from build123d import *

# Parameters (mm, degrees)
F0_W     = 260
F0_H     = 130
F1_DEPTH = 50
F2_R     = 50
F3_DEPTH = 10
F4_W     = 240
F4_H     = 110
F5_DEPTH = 30
F7_DEPTH = 260
F8_R     = 4
F8_R_2   = 4.17612
F9_DEPTH = 25


with BuildPart() as f1:
    # F0 (on Front) → F1 (new body)
    with BuildSketch(Plane.XZ):
        Rectangle(F0_W, F0_H)
    extrude(amount=F1_DEPTH)

    # F2 (on face) → F3 (cut)
    with BuildSketch(Plane(origin=(0, 0, 0), x_dir=(-1, 0, 0), z_dir=(0, 1, 0))):
        with Locations((60, 0)):
            Circle(F2_R)
        with Locations((-60, 0)):
            Circle(F2_R)
    extrude(amount=-F3_DEPTH, mode=Mode.SUBTRACT)

    # F4 (on face) → F5 (cut)
    with BuildSketch(Plane.XZ.offset(50)):
        Rectangle(F4_W, F4_H)
    extrude(amount=-F5_DEPTH, mode=Mode.SUBTRACT)

    # F6 (on face) → F7 (join)
    with BuildSketch(Plane(origin=(-130, 0, 0), x_dir=(0, -1, 0), z_dir=(-1, 0, 0))):
        Polygon((20, -65), (0, -65), (0, -85), (5, -85), (5, -70), (20, -70), align=None)
    extrude(amount=-F7_DEPTH)

    # F8 (on face) → F9 (cut)
    with BuildSketch(Plane(origin=(0, 0, 0), x_dir=(-1, 0, 0), z_dir=(0, 1, 0))):
        with Locations((-72.5, -76.529376)):
            Circle(F8_R)
        with Locations((45.50003, -76.529376)):
            Circle(F8_R_2)
    extrude(amount=-F9_DEPTH, mode=Mode.SUBTRACT)


solid = f1.part
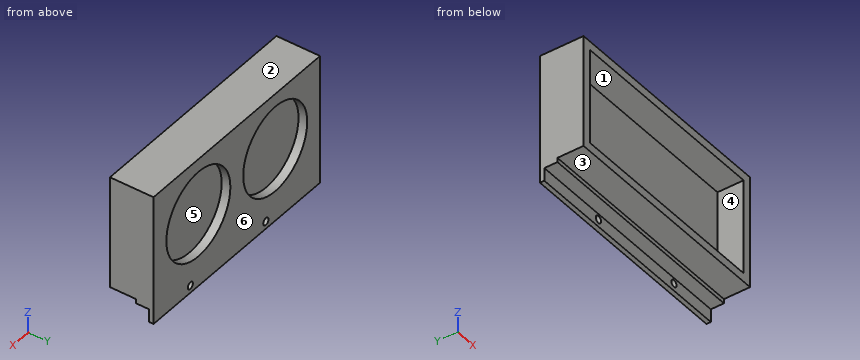
Could you check a few things on this model? Use its own coordinates, in mm. Face numbers are marked on the shaded views. A direction names the side the tool comes from. Give positions to 0.01 mm unless a question says otherwise; leave off trailing zeros. Order: outer loops, then holes, each group sorted by start corner. A loop starts at its lowest first (then second) coordinate and runs counter-clockwise, first axis right, second up.
1. Suppose I cut it at A-A (y = -31.5). Write out the boundary of the cut face in (x, z).
Answers below:
outline: (-130, -65) - (130, -65) - (130, 65) - (-130, 65) - close; hole (-120, -55) - (120, -55) - (120, 55) - (-120, 55) - close
2. For pin 1 (5 mm diameter, centred on x = 60, y = -28.5, fed in from -Z); pin 2 (16.5 mm diameter, centred on x = 28, y = -12.5, fed in from -Z); pin 3 (1.5 mm diameter, centred on x = -45.5, z = -66.5, fed in from -Y); pin 4 (8 mm diameter, centred on x = -62, z = 27, fed in from +Y), each with a flat end and sliding along its axis, tell me the tip position at first contact or that it passes through.
Answers below:
pin 1: stops at z = -65
pin 2: stops at z = -85
pin 3: stops at y = -20
pin 4: stops at y = -10
3. Suppose I cut it at B-B (z = 0). Write out the boundary of the cut face in (x, y).
Answers below:
outline: (-130, -50) - (-120, -50) - (-120, -20) - (120, -20) - (120, -50) - (130, -50) - (130, 0) - (110, 0) - (110, -10) - (10, -10) - (10, 0) - (-10, 0) - (-10, -10) - (-110, -10) - (-110, 0) - (-130, 0) - close
4. I need wall thicknesses on L1, parallel to X at y = -45, z = 15.5; L2, parallel to X at y = -4, z = -37.5; L3, parallel to Z at x = 67, y = -34. Which ranges of each line are inside material? Lowest first, please.
Answers below:
L1: x = -130 to -120, 120 to 130
L2: x = -130 to -93.07, -26.93 to 26.93, 93.07 to 130
L3: z = -65 to -55, 55 to 65
5. Which directions (+Z, -Z, +X, -X, +Y, -Y) give clear straight access to the entire face, cutting with the end or side of a thin tool? Please do the marked faces 4, 5 and 6.
Answers below:
face 4: -Y
face 5: +Y
face 6: +Z, -Z, +X, -X, +Y
6. Suppose I cut it at D-D (x = 71). Write out the boundary of the cut face in (y, z) (3 decimals), plus the area to 3 significant figures.
Answers below:
outline: (-50, -65) - (-20, -65) - (-20, -70) - (-5, -70) - (-5, -72.821) - (0, -72.821) - (0, -48.775) - (-10, -48.775) - (-10, 48.775) - (0, 48.775) - (0, 65) - (-50, 65) - (-50, 55) - (-20, 55) - (-20, -55) - (-50, -55) - close; (-5, -85) - (0, -85) - (0, -80.237) - (-5, -80.237) - close
area: 2,360 mm2
7. Suppose I cut it at C-C (x = -60). Write out the boundary of the cut face in (y, z), plus the area to 4 significant figures.
Answers below:
outline: (-50, -65) - (-20, -65) - (-20, -70) - (-5, -70) - (-5, -85) - (0, -85) - (0, -50) - (-10, -50) - (-10, 50) - (0, 50) - (0, 65) - (-50, 65) - (-50, 55) - (-20, 55) - (-20, -55) - (-50, -55) - close
area: 2,375 mm2
8. Thinking about a two-plate mould opening in Z: for the marked faces 1, 2 and 3, which applies, +Z half, -Z half, draft (parallel to the pull), parting line (faces both ways), or undercut?
Answers below:
face 1: undercut
face 2: +Z half
face 3: -Z half
